The listing builds one solid part. Answer for the finished solid, in the listing's coordinates (mm). A direction names the side the tool comes from. Round coordinates to 2 decimals unless told otherwise and drop trailing zeros. Write each loop counter-clockwise with the first axis right and the second up, starting at its lowest first coordinate (ties: lowest second). Pieces come first, ordered by that corner, then holes. Notation, with made-up numbers: (65.5, 52.5) - (112.5, 52.5) arc R30 cw to (112.5, 83.5) - close; hole circle Ø4 at (-21, -3). An arc over 180 degrees is marked (long way). Return JSON: item names as keys, results as strings. Group by question number.
(1) Each of these flat-tipped pins is pushed along its axis until it touches: pin 1 (5 mm diameter, centred on x = 39.5, z = 46, fed in from -Y) (3 decimals); pin 2 (5.5 mm diameter, centred on y = 0, z = -12.7, fed in from -X); pin 3 (7.5 mm diameter, centred on x = 9.52, z = 46.29, fed in from -Y); pin 4 (4 mm diameter, centred on x = 42.5, y = 90, fed in from +Z). Where does it stop, or does it pass through?
(2) Section D-D, the plane y = 21.5 is taken. Write down the section's boundary in (x, z).
(3) Which of the six approach directions +Z, -Z, +X, -X, +Y, -Y give full straight-line access (tool end or side, diameter ignored) to faces 1 (the cylindrical face through (2.415, 112.314, -19.95)), 2 (the flat face through (22, -3.175, 25)), 3 (the cylindrical face through (42.155, 4.173, -4.946))?
(4) Find the intervals of material crossed by line 1 along Y through (x, z) = (2.4, -12.7); line 2 along Z through (x, y) = (1.7, 0); line 3 along X through (y, z) = (66, -5), in increasing order. Write a range as [from, to].
(5) Determine the mould class of faces 4 (the cylindrical face through (42.11, 108.07, -8.38)), 5 (the cylindrical face through (42.11, 120.03, -10.12)), 6 (the cylindrical face through (42.178, -6.163, -14.231)), 7 (the flat face through (44.526, 60, -9)) for opening direction Y: +Y half, -Y half, draft (parallel to the pull), parting line (faces both ways), or undercut.
(6) Section A-A, the plane z = -12.7 is taken. Write down the section's boundary in (x, y).
(7) Section C-C, the plane x = 21 is taken. Write down the section's boundary in (y, z) (1 decimal).
(8) Section B-B, the plane y = 86.5 is taken. Write down the section's boundary in (x, z), then the cut area to 3 significant figures.
Autodesk Inventor part; units mm, degrees
ref_plane "YZ Plane" through (0, 0, 0) normal (1, 0, 0) x (0, 1, 0)
ref_plane "XZ Plane" through (0, 0, 0) normal (0, 1, 0) x (-1, 0, 0)
ref_plane "XY Plane" through (0, 0, 0) normal (0, 0, 1) x (1, 0, 0)
sketch "Sketch1" plane through (0, 0, 0) normal (1, 0, 0) x (0, 1, 0)
  line L0 (0, 0) -> (127, 0)
  line L1 (127, 0) -> (127, -25.4)
  line L2 (127, -25.4) -> (0, -25.4)
  line L3 (0, -25.4) -> (0, 0)
  line L4 (0, -6.35) -> (0, -19.05)
  line L5 (0, -6.35) -> (76.2, 0)
  line L6 (0, -19.05) -> (76.2, -25.4)
  dimension "d0" = 127
  dimension "d1" = 25.4
  dimension "d18" = 12.7
  dimension "d19" = 6.35
  dimension "d20" = 50.8
  dimension "d21" = 50.8
ref_plane "Work Plane1" through (44.5262, 0, 0) normal (1, 0, 0) x (0, 0, -1)
sketch "Sketch2" plane through (44.5262, 0, 0) normal (1, 0, 0) x (0, 0, -1)
  line L0 (0, 127) -> (0, 0)
  line L1 (0, 0) -> (25.4, 0)
  line L2 (25.4, 0) -> (25.4, 127)
  line L3 (25.4, 127) -> (0, 127)
  line L4 (0, 0) -> (25.4, 0)
  circle A0 centre (12.7, 0) radius 6.35
  dimension "d5" = 25.4
  dimension "d6" = 12.7
  dimension "d7" = 12.7
  dimension "d8" = 0
extrude "Extrusion2" add sketch "Sketch2" against normal blind 44.5262 contours A0 L1 | L1 A0
ref_plane "Work Plane2" through (44.5262, 0, 0) normal (1, 0, 0) x (0, 0, -1)
extrude "Extrusion3" add sketch "Sketch1" along normal blind 44.5262 contours L0 L1 L2 L6 L3 L5
sketch "Sketch4" plane through (0, 0, 0) normal (-1, 0, 0) x (0, 0, 1)
  arc A0 (-19.05, 0) -> (-6.35, 0) centre (-12.7, 0) ccw
  line L0 (0, 76.2) -> (-6.35, 0)
  line L1 (0, 127) -> (0, 76.2)
  line L2 (-25.4, 127) -> (0, 127)
  line L3 (-25.4, 76.2) -> (-25.4, 127)
  line L4 (-19.05, 0) -> (-25.4, 76.2)
  point P0 (0, 0)
hole "Hole2" at (0, 0, -12.7) direction (1, 0, 0) diameter 6.858 end through all
sketch "Sketch5" plane through (0, 0, 0) normal (-1, 0, 0) x (0, 0, 1)
  circle A0 centre (-12.7, 0) radius 3.429
  line L0 (0, 76.2) -> (-6.35, 0)
  line L1 (0, 127) -> (0, 76.2)
  line L2 (-25.4, 127) -> (0, 127)
  line L3 (-25.4, 76.2) -> (-25.4, 127)
  line L4 (-19.05, 0) -> (-25.4, 76.2)
  line L5 (-7.6835, 3.175) -> (55.8165, 3.175)
  line L6 (55.8165, 3.175) -> (55.8165, -3.175)
  line L7 (55.8165, -3.175) -> (-7.6835, -3.175)
  line L8 (-7.6835, -3.175) -> (-7.6835, 3.175)
  arc A1 (-19.05, 0) -> (-6.35, 0) centre (-12.7, 0) ccw
  point P0 (0, 0)
  dimension "d31" = 63.5
  dimension "d32" = 6.35
  dimension "d35" = 127
  dimension "d36" = 123.825
  dimension "d95" = 6.858
  dimension "d96" = 5.0165
extrude "Extrusion4" add sketch "Sketch5" against normal blind 44.5262 contours L5 L6 L7 A1 L0 | L0 A1 L7 L8 L5
sketch "Sketch8" plane through (0, 76.2, -25.4) normal (0, 0, -1) x (-1, 0, 0)
  line L0 (0, 0) -> (0, 50.8)
  line L1 (0, 50.8) -> (-44.5262, 50.8)
  line L2 (-44.5262, 0) -> (-44.5262, 50.8)
  line L3 (0, 0) -> (-44.5262, 0)
  line L4 (0, -76.2) -> (0, 0)
  line L5 (0, 0) -> (-44.5262, 0)
  line L6 (-44.5262, -76.2) -> (-44.5262, 0)
  line L7 (0, 50.8) -> (-44.5262, 50.8)
  line L8 (-39.7637, 50.8) -> (-4.7625, 50.8)
  line L9 (-4.7625, 50.8) -> (-4.7625, -98.425)
  line L10 (-4.7625, -98.425) -> (-39.7637, -98.425)
  line L11 (-39.7637, -98.425) -> (-39.7637, 50.8)
  line L12 (0, -76.2) -> (-44.5262, -76.2)
  point P0 (0, -76.2)
  dimension "d41" = 44.5262
  dimension "d43" = 35.0012
  dimension "d44" = 4.7625
  dimension "d45" = 149.225
extrude "Extrusion5" cut sketch "Sketch8" against normal blind 25.4 contours L9 L12 L11 L3 | L3 L11 L1 L9 | L9 L10 L11 L12
fillet "Fillet1" radius 3.175 2 edges at (39.7637, 0, 0) (4.7625, 0, 0)
fillet "Fillet2" radius 3.175 2 edges at (2.3812, 3.175, -6.0854) (42.1449, 3.175, -6.0854)
sketch "Sketch9" plane through (0, 0, 0) normal (-1, 0, 0) x (0, 0, 1)
  line L0 (0, 76.2) -> (-5.7989, 6.6137)
  line L1 (0, 127) -> (0, 76.2)
  line L2 (-25.4, 127) -> (0, 127)
  line L3 (-25.4, 76.2) -> (-25.4, 127)
  line L4 (-19.05, 0) -> (-25.4, 76.2)
  circle A0 centre (-12.7, 0) radius 3.429
  circle A1 centre (-12.7, 114.8637) radius 8
  line L5 (-19.6282, 118.8637) -> (-5.7718, 118.8637)
  line L6 (-5.7718, 118.8637) -> (-5.7718, 110.8637)
  line L7 (-5.7718, 110.8637) -> (-19.6282, 110.8637)
  line L8 (-19.6282, 110.8637) -> (-19.6282, 118.8637)
  arc A2 (-19.05, 0) -> (-7.2007, -3.175) centre (-12.7, 0) ccw
  line L9 (55.8165, -3.175) -> (-7.2007, -3.175)
  line L10 (55.8165, 3.175) -> (55.8165, -3.175)
  line L11 (-2.6348, 3.175) -> (55.8165, 3.175)
  arc A3 (-5.7989, 6.6137) -> (-2.6348, 3.175) centre (-2.6348, 6.35) ccw
  point P0 (0, 0)
  dimension "d50" = 16
  dimension "d51" = 25.4
  dimension "d52" = 12.7
  dimension "d53" = 8
  dimension "d54" = 4
hole "Hole3" at (0, 118.8637, -19.6282) at (0, 110.8637, -19.6282) at (0, 118.8637, -5.7718) at (0, 110.8637, -5.7718) direction (1, 0, 0) diameter 2.9718 depth 25.4 tip angle 118
sketch "Sketch10" plane through (44.5262, 0, 0) normal (1, 0, 0) x (0, 0, -1)
  line L0 (19.05, 0) -> (25.4, 76.2)
  line L1 (25.4, 76.2) -> (25.4, 127)
  line L2 (25.4, 127) -> (0, 127)
  line L3 (0, 127) -> (0, 76.2)
  line L4 (0, 76.2) -> (5.7989, 6.6137)
  circle A0 centre (12.7, 0) radius 3.429
  circle A1 centre (12.7, 113.546) radius 8
  line L5 (16.7, 106.6178) -> (8.7, 106.6178)
  line L6 (8.7, 106.6178) -> (8.7, 120.4742)
  line L7 (8.7, 120.4742) -> (16.7, 120.4742)
  line L8 (16.7, 120.4742) -> (16.7, 106.6178)
  arc A2 (7.2007, -3.175) -> (19.05, 0) centre (12.7, 0) ccw
  arc A3 (2.6348, 3.175) -> (5.7989, 6.6137) centre (2.6348, 6.35) ccw
  line L9 (2.6348, 3.175) -> (-55.8165, 3.175)
  line L10 (-55.8165, 3.175) -> (-55.8165, -3.175)
  line L11 (-55.8165, -3.175) -> (7.2007, -3.175)
  point P0 (0, 0)
  dimension "d62" = 16
  dimension "d63" = 25.4
  dimension "d64" = 12.7
  dimension "d65" = 8
  dimension "d66" = 4
hole "Hole4" at (44.5262, 106.6178, -16.7) at (44.5262, 106.6178, -8.7) at (44.5262, 120.4742, -8.7) at (44.5262, 120.4742, -16.7) direction (-1, 0, 0) diameter 2.9718 depth 25.4 tip angle 118
sketch "Sketch11" plane through (0, -3.175, -7.2007) normal (0, -1, 0) x (1, 0, 0)
  line L0 (4.7625, 0) -> (4.7625, 4.0257)
  arc A0 (7.9375, 7.2007) -> (4.7625, 4.0257) centre (7.9375, 4.0257) ccw
  line L1 (7.9375, 7.2007) -> (36.5887, 7.2007)
  arc A1 (39.7637, 4.0257) -> (36.5887, 7.2007) centre (36.5887, 4.0257) ccw
  line L2 (39.7637, 4.0257) -> (39.7637, 0)
  line L3 (44.5262, 63.0172) -> (44.5262, 0)
  line L4 (0, 63.0172) -> (44.5262, 63.0172)
  line L5 (0, 63.0172) -> (0, 0)
  line L6 (44.5262, 0) -> (39.7637, 0)
  line L7 (4.7625, 0) -> (0, 0)
  point P0 (0, 7.2007)
  point P1 (9.525, 53.4922)
  dimension "d74" = 9.525
  dimension "d75" = 44.5262
  dimension "d97" = 9.525
hole "Hole5" at (9.525, -3.175, 46.2915) direction (0, 1, 0) diameter 12.7 depth 3.175 tip angle 118
sketch "Sketch12" plane through (44.5262, 0, 0) normal (1, 0, 0) x (0, 0, -1)
  circle A0 centre (8.7, 120.4742) radius 1.4859
  circle A1 centre (16.7, 106.6178) radius 1.4859
  circle A2 centre (8.7, 106.6178) radius 1.4859
  circle A3 centre (16.7, 120.4742) radius 1.4859
  line L0 (19.05, 0) -> (25.4, 76.2)
  line L1 (25.4, 76.2) -> (25.4, 127)
  line L2 (25.4, 127) -> (0, 127)
  line L3 (0, 127) -> (0, 76.2)
  line L4 (0, 76.2) -> (5.7989, 6.6137)
  circle A4 centre (12.7, 0) radius 3.429
  arc A5 (7.2007, -3.175) -> (19.05, 0) centre (12.7, 0) ccw
  arc A6 (2.6348, 3.175) -> (5.7989, 6.6137) centre (2.6348, 6.35) ccw
  line L5 (2.6348, 3.175) -> (-55.8165, 3.175)
  line L6 (-55.8165, 3.175) -> (-55.8165, -3.175)
  line L7 (-55.8165, -3.175) -> (7.2007, -3.175)
  point P0 (0, 0)
  point P1 (12.7, 113.546)
  dimension "d84" = 25.4
  dimension "d85" = 12.7
  dimension "d86" = 13.8564
  dimension "d87" = 6.9282
hole "Hole6" at (44.5262, 113.546, -12.7) direction (-1, 0, 0) diameter 6.35 end through all
equation "\"d19\" = -0.5 * d18 + 0.5 * d1"
equation "\"d21\" = d20"
equation "\"d7\" = 0.5 * d5"
equation "\"d36\" = d35 - 0.5 * d32"
equation "\"d44\" = -0.5 * d43 + 0.5 * d41"
equation "\"d52\" = 0.5 * d51"
equation "\"d54\" = 0.5 * d53"
equation "\"d64\" = 0.5 * d63"
equation "\"d66\" = 0.5 * d65"
properties part number "WheelIntakeMount3.0"
Working result:
{
 "1": {"pin 1": "stops at y = -3.175", "pin 2": "passes through", "pin 3": "stops at y = 1.56", "pin 4": "stops at z = 0"},
 "2": {"outline": "(0, -20.84) - (4.76, -20.84) - (4.76, -4.56) - (0, -4.56) - close; (39.76, -20.84) - (44.53, -20.84) - (44.53, -4.56) - (39.76, -4.56) - close"},
 "3": {"face 1": "-X", "face 2": "+Z, +X, -X, -Y", "face 3": "+Z, +X, -X"},
 "4": {"line 1": "y = [-6.35, -3.43], [3.43, 110.37], [116.72, 127]", "line 2": "z = [-19.05, -16.13], [-9.27, 55.82]", "line 3": "x = [0, 4.76], [39.76, 44.53]"},
 "5": {"face 4": "undercut", "face 5": "undercut", "face 6": "-Y half", "face 7": "draft"},
 "6": {"outline": "(0, -6.35) - (4.76, -6.35) - (4.76, -3.43) - (0, -3.43) - close; (0, 3.43) - (4.76, 3.43) - (4.76, 110.37) - (0, 110.37) - close; (0, 116.72) - (4.76, 116.72) - (4.76, 127) - (0, 127) - close; (39.76, -6.35) - (44.53, -6.35) - (44.53, -3.43) - (39.76, -3.43) - close; (39.76, 3.43) - (44.53, 3.43) - (44.53, 110.37) - (39.76, 110.37) - close; (39.76, 116.72) - (44.53, 116.72) - (44.53, 127) - (39.76, 127) - close"},
 "7": {"outline": "(-3.2, 0) - (3.2, 0) - (3.2, 55.8) - (-3.2, 55.8) - close"},
 "8": {"outline": "(0, -25.4) - (4.76, -25.4) - (4.76, 0) - (0, 0) - close; (39.76, -25.4) - (44.53, -25.4) - (44.53, 0) - (39.76, 0) - close", "area": "242 mm^2"}
}
